```python
from build123d import *

# Parameters (mm, degrees)
SKETCH_1_R      = 10.15
SKETCH_1_R_2    = 2.65
EXTRUDE_1_DEPTH = 4
FILLET_1_R      = 10


with BuildPart() as part:
    # 草图1 → 凸台-拉伸1 (new body)
    with BuildSketch(Plane.XY):
        with BuildLine():
            Line((-10, 70), (-10, 22.912878475))
            ThreePointArc((-10, 22.912878475), (0, -25), (10, 22.912878475))
            Line((10, 22.912878475), (10, 70))
            Line((10, 70), (-10, 70))
        make_face()
        Circle(SKETCH_1_R, mode=Mode.SUBTRACT)
        with Locations((0, 21)):
            Circle(SKETCH_1_R_2, mode=Mode.SUBTRACT)
        with Locations((18.186533479, -10.5)):
            Circle(SKETCH_1_R_2, mode=Mode.SUBTRACT)
        with Locations((-18.186533479, -10.5)):
            Circle(SKETCH_1_R_2, mode=Mode.SUBTRACT)
        with Locations((0, 60)):
            Circle(SKETCH_1_R_2, mode=Mode.SUBTRACT)
        with Locations((0, 35)):
            Circle(SKETCH_1_R_2, mode=Mode.SUBTRACT)
        with Locations((0, 47.5)):
            Circle(SKETCH_1_R_2, mode=Mode.SUBTRACT)
    extrude(amount=EXTRUDE_1_DEPTH)

    # 圆角1
    fillet_1_edges = [part.edges().sort_by_distance(p)[0] for p in [
        (10, 22.912878475, 2),
        (10, 70, 2),
        (-10, 70, 2),
        (-10, 22.912878475, 2),
    ]]
    fillet(fillet_1_edges, radius=FILLET_1_R - 0.0001)  # a hair under: the kernel refuses the full size


solid = part.part
```
Model file for the job. Use its own axes, mm. A direction names the side the tool comes from. Round coordinates to 2 decimals unless told otherwise and drop trailing zeros. Loops run counter-clockwise (first coordinate to the right, second up) from the corner with the lowest first, then second, coordinate; pieces in that order, holes last. Notation, with made-up numbers: M 66.5,-24 L 86.5,-24 A29 ccw 86.5,4 Z; hole C 61.25,-1 d6. An arc over 180 degrees is marked long. Put each result on its own line as item: value. Start each with the question number.
Item 1: 3-axis set-ups, long thin cutter, end or side, ignore diameter. For faces 4 (the face through (-0.886, -24.984, 1.972)), 5 (the face through (-10, 45, 2)): which of +Z, -Z, +X, -X, +Y, -Y reach the whole face in a straight line?
Item 2: Cut at A-A (z = 2.7). Give the number of separate pieces and of enclosed holes in the cut face, then the cut area to 3 significant figures.
Item 3: Drill centre lines: line 1 along Y through (x, z) = (0, 1.05); line 2 along X through (y, z) = (-11, 3.6); line 3 along X through (y, z) = (53, 2.2). Where is each one in solid material? Low to high.
Item 4: Cut at B-B (x = -17). List the corners of the cut face in (y, z).
Item 5: Drop flat-ended pins along their axis: P1, Ø16, axis at x = 0, y = 0, coming from the -Z side; P2, Ø2, axis at x = -5.5, z = 2.5, coming from the +Y side; P3, Ø1.5, axis at x = -7, z = 2, coming from the -Y side; P4, Ø2, axis at y = 37, z = 2.5, coming from the -X side. Give the stop position or say it passes through.
Item 6: Cut at D-D (x = 1.5). List the corners of the cut face in (y, z), then the cut area to 3 significant figures.
Item 7: Mould opens along X. For faces 1 (the face through (-16, -12, 2)), 2 (the face through (-7.15, 66.99, 2.03)), 3 (the face through (10, 44, 2)) say: released by +X, released by -X, zero draft, split by the parting line, or undercut.
Item 8: Cut at C-C (y = 47.5). List the corners of the cut face in (x, z).
Answer block:
1. face 4: +Z, -Z
1. face 5: +Z, -Z, -X, +Y
2. separate pieces: 1
2. enclosed holes: 7
2. area: 2,390 mm2
3. line 1: -25 to -10.15, 10.15 to 18.35, 23.65 to 32.35, 37.65 to 44.85, 50.15 to 57.35, 62.65 to 70
3. line 2: -22.45 to -20.79, -15.58 to 15.58, 20.79 to 22.45
3. line 3: -10 to 10
4. outline: M -18.33,0 L -12.87,0 L -12.87,4 L -18.33,4 Z; M -8.13,0 L 18.33,0 L 18.33,4 L -8.13,4 Z
5. P1: through
5. P2: y = 68.93
5. P3: y = -24.21
5. P4: x = -10
6. outline: M -24.95,0 L -10.04,0 L -10.04,4 L -24.95,4 Z; M 10.04,0 L 18.82,0 L 18.82,4 L 10.04,4 Z; M 23.18,0 L 32.82,0 L 32.82,4 L 23.18,4 Z; M 37.18,0 L 45.32,0 L 45.32,4 L 37.18,4 Z; M 49.68,0 L 57.82,0 L 57.82,4 L 49.68,4 Z; M 62.18,0 L 69.89,0 L 69.89,4 L 62.18,4 Z
6. area: 229 mm2
7. face 1: undercut
7. face 2: released by -X
7. face 3: released by +X
8. outline: M -10,0 L -2.65,0 L -2.65,4 L -10,4 Z; M 2.65,0 L 10,0 L 10,4 L 2.65,4 Z
